Read the model definition and answer for the solid it produces. Units are mm, in the model's axes. Round coordinates to 2 decimals unless told otherwise and drop trailing zeros. Order: outer loops, then holes, each group sorted by start corner. A loop starts at its lowest first (then second) coordinate and runs counter-clockwise, first axis right, second up. Notation, with made-up numbers: M -28.5,64.25 L -14.5,64.25 A13 ccw -14.5,75.25 Z; hole C 27,27 d2. An arc over 180 degrees is marked long. Use one line per item in the form item = value. Start each with the question number.
from build123d import *

# Parameters (mm, degrees)
SKETCH1_W           = 53
SKETCH1_H           = 35
BOSS_EXTRUDE1_DEPTH = 10
SKETCH2_R           = 2
SKETCH2_R_2         = 9.699233374
CUT_EXTRUDE1_DEPTH  = 11


with BuildPart() as part:
    # Sketch1 → Boss-Extrude1 (new body)
    with BuildSketch(Plane(origin=(0, 0, 0), x_dir=(1, 0, 0), z_dir=(0, 1, 0))):
        Rectangle(SKETCH1_W, SKETCH1_H)
    extrude(amount=BOSS_EXTRUDE1_DEPTH)

    # Sketch2 → Cut-Extrude1 (cut, through all)
    with BuildSketch(Plane(origin=(0, 10, 0), x_dir=(1, 0, 0), z_dir=(0, 1, 0))):
        with Locations((-17.5, 15)):
            Circle(SKETCH2_R)
        with Locations((17.5, 15)):
            Circle(SKETCH2_R)
        with Locations((-17.5, -15)):
            Circle(SKETCH2_R)
        with Locations((17.5, -15)):
            Circle(SKETCH2_R)
        Circle(SKETCH2_R_2)
    extrude(amount=-CUT_EXTRUDE1_DEPTH, mode=Mode.SUBTRACT)


solid = part.part
Item 1: Find the intervals of material crossed by L1, parallel to Z at x = 17.5, y = 4.5; L2, parallel to Z at x = -0.5, y = 1.5; L3, parallel to Z at x = -19, y = 5, in increasing order. Write a range as [from, to].
Item 2: Section C-C (y = 8.75) is taken. Write down the section's boundary in (x, z).
Item 3: For a pull along Z with two mould halves and no side action, classify faces 1 (the flat face through (-6, 10, -8)), 2 (the flat face through (0, 5, -17.5)), 3 (the cylindrical face through (17.24, 5.07, -16.983)) as pulls with the +Z half, pulls with the -Z half, needs draft (parallel to the pull), parting line crosses it, or undercut.
Item 4: Section B-B (x = 17.5) is taken. Write down the section's boundary in (y, z), and give its area (3 significant figures).
Item 5: Section A-A (z = 0) is taken. Write down the section's boundary in (x, y).
Item 6: Section D-D (z = -15) is taken. Write down the section's boundary in (x, y), and give its area (3 significant figures).
The answers:
q1.L1 = [-17.5, -17], [-13, 13], [17, 17.5]
q1.L2 = [-17.5, -9.69], [9.69, 17.5]
q1.L3 = [-17.5, -16.32], [-13.68, 13.68], [16.32, 17.5]
q2.outline = M -26.5,-17.5 L 26.5,-17.5 L 26.5,17.5 L -26.5,17.5 Z; hole C -17.5,-15 d4; hole C -17.5,15 d4; hole C 0,0 d19.4; hole C 17.5,-15 d4; hole C 17.5,15 d4
q3.face_1 = needs draft
q3.face_2 = pulls with the -Z half
q3.face_3 = undercut
q4.outline = M 0,-17.5 L 10,-17.5 L 10,-17 L 0,-17 Z; M 0,-13 L 10,-13 L 10,13 L 0,13 Z; M 0,17 L 10,17 L 10,17.5 L 0,17.5 Z
q4.area = 270 mm²
q5.outline = M -26.5,0 L -9.7,0 L -9.7,10 L -26.5,10 Z; M 9.7,0 L 26.5,0 L 26.5,10 L 9.7,10 Z
q6.outline = M -26.5,0 L -19.5,0 L -19.5,10 L -26.5,10 Z; M -15.5,0 L 15.5,0 L 15.5,10 L -15.5,10 Z; M 19.5,0 L 26.5,0 L 26.5,10 L 19.5,10 Z
q6.area = 450 mm²
